Check sheet for the modelled part. Datum: model origin and axes. Units: mm. Round coordinates to 2 decimals unless told otherwise and drop trailing zeros. Loops run counter-clockwise (first coordinate to the right, second up) from the corner with the lowest first, then second, coordinate; pieces in that order, holes last. Notation, with made-up numbers: M 86.5,54 L 129.5,54 A21 cw 129.5,85 Z; hole C -37,12 d1. An arc over 180 degrees is marked long. One line per question, with ' | ' between items. Start each with the question number.
(1) Section check A-A (y = -97). Record the boundary of the cut face in (x, z).
(2) Section check B-B (x = 828.5). Record the boundary of the cut face in (y, z).
(3) Go/stop test with flat-tipped pins: P1, Ø0.5, axis at x = -604.5, z = -0.5, coming from the -Y side; P2, Ø0.5, axis at x = 194.5, z = -0.5, coming from the +Y side. Record where each tip stops, or that it passes through.
(4) Section check C-C (z = -0.4). Count the separate pieces of the cut face and the enclosed holes in it, and give its area (3 significant figures).
(5) Thickness scan on probe 1 along X at (y, z) = (-553, -0.8); probe 2 along Y at (x, z) = (577.5, -0.4); probe 3 along Y at (x, z) = (-226, -0.6). Record the ranges inside material, lowest first. Write a range as [from, to].
```python
from build123d import *

# Parameters (mm, degrees)
CROQUIS1_W            = 1652
CROQUIS1_H            = 800
BRIDA_BASE1_DEPTH     = 1
CROQUIS14_W           = 51.8
CROQUIS14_H           = 50.8
CROQUIS14_W_2         = 50.8
CORTAR_EXTRUIR1_DEPTH = 1219.148680595
REDONDEO1_R           = 10
REDONDEO2_R           = 10
CROQUIS17_W           = 370
CROQUIS17_H           = 160
CROQUIS17_W_2         = 5
CROQUIS17_H_2         = 30
CROQUIS17_R           = 6.1
CORTAR_EXTRUIR2_DEPTH = 10
REDONDEO3_R           = 50
REDONDEO4_R           = 20
CROQUIS18_R           = 10
CROQUIS18_W           = 51.8
CROQUIS18_H           = 51.8
CROQUIS18_W_2         = 102.1
CROQUIS18_H_2         = 102.1
CORTAR_EXTRUIR3_DEPTH = 10
REDONDEO5_R           = 10
REDONDEO6_R           = 20
REDONDEO7_R           = 10


# Sheet-metal steps are written as plain solids
with BuildPart() as part:
    # Brida base1: sheet metal written as solids
    # Croquis1 → Brida base1 (new body)
    with BuildSketch(Plane.XY):
        with Locations((191.278244715, -270.097142857)):
            Rectangle(CROQUIS1_W, CROQUIS1_H)
    extrude(amount=-BRIDA_BASE1_DEPTH)

    # Croquis14 → Cortar-Extruir1 (cut, through all)
    with BuildSketch(Plane.XY.offset(-1)):
        with Locations((-608.821755285, -199.597142857)):
            Rectangle(CROQUIS14_W, CROQUIS14_H)
        with Locations((991.878244715, -199.597142857)):
            Rectangle(CROQUIS14_W_2, CROQUIS14_H)
        with Locations((591.378244715, -199.597142857)):
            Rectangle(CROQUIS14_W, CROQUIS14_H)
        Polygon((617.278244715, 81.002857143), (617.278244715, 131.802857143), (565.478244715, 131.802857143), (565.478244715, 81.002857143), (591.378244715, 81.002857143), align=None)
        Polygon((617.278244715, 131.802857143), (1017.278244715, -174.197142857), (1017.278244715, 131.802857143), align=None)
        with Locations((-207.621755285, -199.597142857)):
            Rectangle(CROQUIS14_W, CROQUIS14_H)
        with Locations((192.378244715, -199.597142857)):
            Rectangle(CROQUIS14_W, CROQUIS14_H)
        with Locations((191.311578048, 106.402857143)):
            Rectangle(CROQUIS14_W, CROQUIS14_H)
        with Locations((-208.755088618, 106.402857143)):
            Rectangle(CROQUIS14_W, CROQUIS14_H)
        with Locations((-608.821755285, 106.402857143)):
            Rectangle(CROQUIS14_W, CROQUIS14_H)
    extrude(amount=CORTAR_EXTRUIR1_DEPTH, mode=Mode.SUBTRACT)

    # Redondeo1
    redondeo1_edges = [part.edges().sort_by_distance(p)[0] for p in [
        (617.278244715, -224.997142857, -0.5),
    ]]
    fillet(redondeo1_edges, radius=REDONDEO1_R)

    # Redondeo2
    redondeo2_edges = [part.edges().sort_by_distance(p)[0] for p in [
        (-582.921755285, -174.197142857, -0.5),
        (-582.921755285, -224.997142857, -0.5),
        (-181.721755285, -174.197142857, -0.5),
        (-233.521755285, -174.197142857, -0.5),
        (-233.521755285, -224.997142857, -0.5),
        (-181.721755285, -224.997142857, -0.5),
        (166.478244715, -174.197142857, -0.5),
        (166.478244715, -224.997142857, -0.5),
        (218.278244715, -224.997142857, -0.5),
        (218.278244715, -174.197142857, -0.5),
        (617.278244715, -174.197142857, -0.5),
        (565.478244715, -174.197142857, -0.5),
        (565.478244715, -224.997142857, -0.5),
        (966.478244715, -224.997142857, -0.5),
        (966.478244715, -174.197142857, -0.5),
        (565.478244715, 81.002857143, -0.5),
        (617.278244715, 81.002857143, -0.5),
        (-582.921755285, 81.002857143, -0.5),
        (-234.655088618, 81.002857143, -0.5),
        (-182.855088618, 81.002857143, -0.5),
        (165.411578048, 81.002857143, -0.5),
        (217.211578048, 81.002857143, -0.5),
    ]]
    fillet(redondeo2_edges, radius=REDONDEO2_R)

    # Croquis17 → Cortar-Extruir2 (cut)
    with BuildSketch(Plane(origin=(0, 0, -1), x_dir=(-1, 0, 0), z_dir=(0, 0, -1))):
        with Locations((449.721755285, -590.097142857)):
            Rectangle(CROQUIS17_W, CROQUIS17_H)
        with Locations((632.221755285, -495.097142857)):
            Rectangle(CROQUIS17_W_2, CROQUIS17_H_2)
        with Locations((609.321755285, -495.097142857)):
            Circle(CROQUIS17_R)
    extrude(amount=-CORTAR_EXTRUIR2_DEPTH, mode=Mode.SUBTRACT)

    # Redondeo3
    redondeo3_edges = [part.edges().sort_by_distance(p)[0] for p in [
        (-264.721755285, -670.097142857, -0.5),
        (1017.278244715, -670.097142857, -0.5),
    ]]
    fillet(redondeo3_edges, radius=REDONDEO3_R)

    # Redondeo4
    # the kernel refuses this fillet: 20 mm, written as the material it adds along each edge
    with BuildSketch(Plane(origin=(-264.721755285, -510.097142857, -1), x_dir=(0, -1, 0), z_dir=(0, 0, 1))) as redondeo4_piece_1:
        with BuildLine():
            CenterArc((REDONDEO4_R, -REDONDEO4_R), REDONDEO4_R, 90, 90)
            Line((0, -REDONDEO4_R), (0, 0))
            Line((0, 0), (REDONDEO4_R, 0))
        make_face()
    extrude(amount=1)
    # the kernel refuses this fillet: 20 mm, written as the material it takes off along each edge
    with BuildSketch(Plane(origin=(-629.721755285, -510.097142857, -51), x_dir=(1, 0, 0), z_dir=(0, 0, 1))) as redondeo4_2_piece_1:
        with BuildLine():
            CenterArc((REDONDEO4_R, REDONDEO4_R), REDONDEO4_R, 180, 90)
            Line((0, REDONDEO4_R), (0, 0))
            Line((0, 0), (REDONDEO4_R, 0))
        make_face()
    extrude(amount=101, mode=Mode.SUBTRACT)
    with BuildSketch(Plane(origin=(-634.721755285, -480.097142857, -34.071891388), x_dir=(1, 0, 0), z_dir=(0, 0, 1))) as redondeo4_2_piece_2:
        with BuildLine():
            CenterArc((20, 13.228756555), REDONDEO4_R, 180, 41.409622109)
            Line((0, 13.228756555), (0, 0))
            Line((0, 0), (5, 0))
        make_face()
    extrude(amount=67.143782777, mode=Mode.SUBTRACT)

    # Croquis18 → Cortar-Extruir3 (cut)
    with BuildSketch(Plane(origin=(0, 0, -1), x_dir=(-1, 0, 0), z_dir=(0, 0, -1))):
        with Locations((214.721755285, -620.097142857)):
            Circle(CROQUIS18_R)
        with Locations((609.321755285, -443.737142857)):
            Rectangle(CROQUIS18_W, CROQUIS18_H)
        with Locations((-591.378244715, -554.697142857)):
            Rectangle(CROQUIS18_W, CROQUIS18_H)
        with Locations((-966.228244715, -619.047142857)):
            Rectangle(CROQUIS18_W_2, CROQUIS18_H_2)
        with Locations((214.721755285, -554.697142857)):
            Rectangle(CROQUIS18_W, CROQUIS18_H)
    extrude(amount=-CORTAR_EXTRUIR3_DEPTH, mode=Mode.SUBTRACT)

    # Redondeo5
    redondeo5_edges = [part.edges().sort_by_distance(p)[0] for p in [
        (565.478244715, -528.797142857, -0.5),
        (565.478244715, -580.597142857, -0.5),
        (617.278244715, -580.597142857, -0.5),
        (617.278244715, -528.797142857, -0.5),
        (915.178244715, -567.997142857, -0.5),
        (-188.821755285, -528.797142857, -0.5),
        (-240.621755285, -528.797142857, -0.5),
        (-240.621755285, -580.597142857, -0.5),
        (-188.821755285, -580.597142857, -0.5),
    ]]
    fillet(redondeo5_edges, radius=REDONDEO5_R)

    # Redondeo6
    redondeo6_edges = [part.edges().sort_by_distance(p)[0] for p in [
        (-629.721755285, -480.097142857, -0.5),
    ]]
    fillet(redondeo6_edges, radius=REDONDEO6_R)

    # Redondeo7
    redondeo7_edges = [part.edges().sort_by_distance(p)[0] for p in [
        (-583.421755285, -469.637142857, -0.5),
        (-583.421755285, -417.837142857, -0.5),
    ]]
    fillet(redondeo7_edges, radius=REDONDEO7_R)


solid = part.part
```
The answers:
1) outline: M -634.72,-1 L 916.37,-1 L 916.37,0 L -634.72,0 Z
2) outline: M -670.1,-1 L -29.78,-1 L -29.78,0 L -670.1,0 Z
3) P1: y = -510.1 | P2: y = 81
4) separate pieces: 1 | enclosed holes: 7 | area: 1,160,000 mm²
5) probe 1: [-264.72, -240.62], [-188.82, 565.48], [617.28, 1017.28] | probe 2: [-670.1, -580.6], [-528.8, -225], [-174.2, 81] | probe 3: [-668.81, -580.6], [-528.8, -224.69], [-174.51, 81.09]
